```python
from build123d import *

# Parameters (mm, degrees)
SKETCH1_R           = 3.5
SKETCH1_W           = 13
SKETCH1_H           = 19.3
BOSS_EXTRUDE1_DEPTH = 3


with BuildPart() as part:
    # Sketch1 → Boss-Extrude1 (new body)
    with BuildSketch(Plane(origin=(0, 0, 0), x_dir=(1, 0, 0), z_dir=(0, 1, 0))):
        Polygon((7, 20), (10, 20), (10, -20), (7, -20), (7, -23), (-7, -23), (-7, -20), (-10, -20), (-10, 20), (-7, 20), (-7, 23), (7, 23), align=None)
        with Locations((0, -13.5)):
            Circle(SKETCH1_R, mode=Mode.SUBTRACT)
        with Locations((0, 4.15)):
            Rectangle(SKETCH1_W, SKETCH1_H, mode=Mode.SUBTRACT)
    extrude(amount=BOSS_EXTRUDE1_DEPTH)


solid = part.part
```
Geometry check sheet. Reference: the model listing, model coordinates, mm. A direction names the side the tool comes from. Give positions to 0.01 mm unless a question says otherwise; leave off trailing zeros. Order: outer loops, then holes, each group sorted by start corner. A loop starts at its lowest first (then second) coordinate and runs counter-clockwise, first axis right, second up. Notation, with made-up numbers: (16.25, -14.75) -> (53.25, -14.75) arc R32 cw to (53.25, 11.25) -> close; hole circle Ø4 at (82, 21). An arc over 180 degrees is marked (long way). Write each question's results on one line, items separated by ' | '. Start each with the question number.
(1) Access from +Z, -Z, +X, -X, +Y, -Y to the whole of each face (thin tool, end or side, straight path). Record for faces 5 (the face through (8, 1, -20)), 6 (the face through (9, 1, 20)), 7 (the face through (-9, 1, -20)), 8 (the face through (-8, 1, 20)).
(2) Scan lines: line 1 (X direction, y = 1.2, z = -3); line 2 (Z direction, x = -5, y = 0.5); line 3 (Z direction, x = -1.75, y = 0.5). Record each from-to range of solid material in increasing order.
(3) Sectioned sample at A-A (z = 13.5). Enter the section's corners in (x, y), plus the area to 3 significant figures.
(4) Sectioned sample at D-D (x = -5.5). Enter the section's corners in (y, z).
(5) Sectioned sample at C-C (y = 1.2). Enter the section's corners in (x, z).
(6) Mould release check, pull along Z, two halves, no side actions. Record for faces 1 (the face through (0, 1, -23)), 2 (the face through (0, 1, 23)), 3 (the face through (6.5, 1, -4)), 4 (the face through (7, 1, 21)): pulls with the +Z half, pulls with the -Z half, needs draft (parallel to the pull), parting line crosses it, or undercut.
(7) Sectioned sample at B-B (x = 0). Enter the section's corners in (y, z), plus the area to 3 significant figures.
(8) Gauge pin test, flat ends, axial feed: P1, Ø2, axis at x = -4, z = -6.5, coming from the -Y side; P2, Ø1.5, axis at y = 1.5, z = -21.5, coming from the +X side; P3, Ø11, axis at x = 0, z = 13.5, coming from the +Y side; P4, Ø1.5, axis at x = -8, y = 1.5, coming from the -Z side. Record the tip position at first contact, or that the pin passes through.
Answer below:
1) face 5: -Z, +X, +Y, -Y | face 6: +Z, +X, +Y, -Y | face 7: -Z, -X, +Y, -Y | face 8: +Z, -X, +Y, -Y
2) line 1: -10 to -6.5, 6.5 to 10 | line 2: -23 to -13.8, 5.5 to 23 | line 3: -23 to -13.8, 5.5 to 10.47, 16.53 to 23
3) outline: (-10, 0) -> (-3.5, 0) -> (-3.5, 3) -> (-10, 3) -> close; (3.5, 0) -> (10, 0) -> (10, 3) -> (3.5, 3) -> close | area: 39.0 mm2
4) outline: (0, -23) -> (3, -23) -> (3, -13.8) -> (0, -13.8) -> close; (0, 5.5) -> (3, 5.5) -> (3, 23) -> (0, 23) -> close
5) outline: (-10, -20) -> (-7, -20) -> (-7, -23) -> (7, -23) -> (7, -20) -> (10, -20) -> (10, 20) -> (7, 20) -> (7, 23) -> (-7, 23) -> (-7, 20) -> (-10, 20) -> close; hole (-6.5, -13.8) -> (6.5, -13.8) -> (6.5, 5.5) -> (-6.5, 5.5) -> close; hole circle Ø7 at (0, 13.5)
6) face 1: pulls with the -Z half | face 2: pulls with the +Z half | face 3: undercut | face 4: needs draft
7) outline: (0, -23) -> (3, -23) -> (3, -13.8) -> (0, -13.8) -> close; (0, 5.5) -> (3, 5.5) -> (3, 10) -> (0, 10) -> close; (0, 17) -> (3, 17) -> (3, 23) -> (0, 23) -> close | area: 59.1 mm2
8) P1: through | P2: x = 7 | P3: y = 3 | P4: z = -20
